Geometry check sheet. Reference: the model listing, model coordinates, mm. A direction names the side the tool comes from. Coordinates: 2 decimals unless noted, no trailing zeros. Order: outer loops, then holes, each group sorted by start corner. A loop starts at its lowest first (then second) coordinate and runs counter-clockwise, first axis right, second up. Notation, with made-up numbers: (8, 19.25) - (17, 19.25) arc R9 cw to (17, 23.25) - close; hole circle Ø5 at (84.5, -23.75). An arc over 180 degrees is marked (long way). Use CSV: the item, a comma, the result in double quotes. Start each with the question number.
1) Sectioned sample at C-C, the plane x = 58. Record the cut outline in (y, z).
2) Draft check along X on faces 1 (the flat face through (-100, 613, -231)), 2 (the flat face through (-126, 0, 157)), 3 (the flat face through (30, 547, 218)), 4 (the flat face through (97.679, 613, -231)). Enter one of: released by +X, released by -X, zero draft, split by the parting line, or undercut.
3) Sectioned sample at A-A, the plane z = 0. Record the cut outline in (x, y), and give its area (3 significant figures).
4) Depth check by flat-ended pin: P1, Ø2, axis at x = -98.5, z = -124.5, coming from the -Y side; P2, Ø6, axis at x = 112, y = 822, coming from the -Z side; P3, Ø10, axis at y = 637.5, z = -81.5, coming from the -X side. Enter the tip coordinate at first touch or a pass-through.
5) Tool access check on faces 5 (the cylindrical face through (-199.96, 547.23, -3.98)), 6 (the flat face through (-3, 1210, -5)), 7 (the flat face through (0, 547, -220)). Record the directions out of +Z, -Z, +X, -X, +Y, -Y that give a thin tool (end or side, any length) a straight path to the whole face; none if there is none.
6) Sectioned sample at B-B, the plane y = 532. Record the cut outline in (x, z), and give its area (3 significant figures).
7) Thickness scan on probe 1 along X at (y, z) = (138, -219.5); probe 2 along Z at (x, y) = (-110, 535); probe 3 along Y at (x, z) = (-63.5, 108). Record the ranges inside material, lowest first. Write a range as [from, to].
from build123d import *

# Parameters (mm, degrees)
BOSS_EXTRUDE1_DEPTH = 1110
SKETCH2_R           = 240
BOSS_EXTRUDE2_DEPTH = 100
BOSS_EXTRUDE3_DEPTH = 1210


with BuildPart() as part:
    # Sketch1 → Boss-Extrude1 (new body)
    with BuildSketch(Plane(origin=(0, 0, 0), x_dir=(1, 0, 0), z_dir=(0, 1, 0))):
        with BuildLine():
            Line((-30, -197.737199333), (-30, -238.117617996))
            ThreePointArc((-30, -238.117617996), (0, 240), (30, -238.117617996))
            Line((30, -238.117617996), (30, -197.737199333))
            ThreePointArc((30, -197.737199333), (200, 0), (30, 197.737199333))
            Line((30, 197.737199333), (30, 220))
            Line((30, 220), (-30, 220))
            Line((-30, 220), (-30, 197.737199333))
            ThreePointArc((-30, 197.737199333), (-200, 0), (-30, -197.737199333))
        make_face()
    extrude(amount=BOSS_EXTRUDE1_DEPTH)

    # Sketch2 → Boss-Extrude2 (add)
    with BuildSketch(Plane(origin=(0, 1110, 0), x_dir=(1, 0, 0), z_dir=(0, 1, 0))):
        with Locations(Location((0, 0, 0), (0, 0, 262.819244219))):
            Circle(SKETCH2_R)
    extrude(amount=BOSS_EXTRUDE2_DEPTH)

    # Sketch3 → Boss-Extrude3 (add, through all)
    with BuildSketch(Plane(origin=(0, 1210, 0), x_dir=(1, 0, 0), z_dir=(0, 1, 0))):
        with BuildLine():
            Line((-100, 242.859479034), (-100, 240))
            Line((-100, 240), (-100, 218.174242293))
            ThreePointArc((-100, 218.174242293), (-51.177054673, 234.48008247), (-3e-09, 240))
            ThreePointArc((-3e-09, 240), (-50.020437376, 240.715015829), (-100, 242.859479034))
        make_face()
        with BuildLine():
            ThreePointArc((97.679334818, 242.72819872), (48.858713445, 240.682182644), (-3e-09, 240))
            ThreePointArc((-3e-09, 240), (49.932288955, 234.748304615), (97.679334818, 219.223054329))
            Line((97.679334818, 219.223054329), (97.679334818, 242.72819872))
        make_face()
    extrude(amount=-BOSS_EXTRUDE3_DEPTH)


solid = part.part
Evaluation:
1,outline,"(0, -240.96) - (1210, -240.96) - (1210, 232.89) - (0, 232.89) - (0, 191.41) - (1110, 191.41) - (1110, -191.41) - (0, -191.41) - close"
2,face 1,"released by -X"
2,face 2,"zero draft"
2,face 3,"undercut"
2,face 4,"released by +X"
3,outline,"(-240, 0) - (-200, 0) - (-200, 1110) - (200, 1110) - (200, 0) - (240, 0) - (240, 1210) - (-240, 1210) - close"
3,area,"137,000 mm²"
4,P1,"y = 1110"
4,P2,"z = -213.82"
4,P3,"x = -227.48"
5,face 5,"-Y"
5,face 6,"+Z, -Z, +X, -X, +Y"
5,face 7,"+Z, -Y"
6,outline,"(-100, -242.86) arc R1750 cw to (0, -240) arc R1750 cw to (97.68, -242.73) - (97.68, -219.22) arc R240 ccw to (30, 238.12) - (30, 197.74) arc R200 cw to (30, -197.74) - (30, -220) - (-30, -220) - (-30, -197.74) arc R200 cw to (-30, 197.74) - (-30, 238.12) arc R240 ccw to (-100, -218.17) - close"
6,area,"53,200 mm²"
7,probe 1,"[-100, -30], [30, 97.68]"
7,probe 2,"[-213.31, -167.03], [167.03, 213.31]"
7,probe 3,"[1110, 1210]"
